```python
from build123d import *

# Parameters (mm, degrees)
SKETCH1_R                 = 9.5377
BOSS_EXTRUDE1_DEPTH       = 29.591
SKETCH2_R                 = 3.81
BOSS_EXTRUDE2_DEPTH       = 10.16
SKETCH3_R                 = 1.9939
CUT_EXTRUDE1_DEPTH        = 12.7
SKETCH4_R                 = 8.4836
CUT_EXTRUDE2_DEPTH        = 27.94
FILLET1_R                 = 3.81
F_4_48_TAPPED_HOLE2_D     = 2.3749
F_4_48_TAPPED_HOLE2_DEPTH = 8.89
F_4_48_TAPPED_HOLE2_TIP   = 0.713491942


with BuildPart() as part:
    # Sketch1 → Boss-Extrude1 (new body)
    with BuildSketch(Plane(origin=(0, 0, 0), x_dir=(1, 0, 0), z_dir=(0, 1, 0))):
        with Locations(Location((0, 0, 0), (0, 0, 90))):
            Circle(SKETCH1_R)
    extrude(amount=BOSS_EXTRUDE1_DEPTH)

    # Sketch2 → Boss-Extrude2 (add)
    with BuildSketch(Plane(origin=(0, 29.591, 0), x_dir=(1, 0, 0), z_dir=(0, 1, 0))):
        with Locations(Location((0, 0, 0), (0, 0, 270))):
            Circle(SKETCH2_R)
    extrude(amount=BOSS_EXTRUDE2_DEPTH)

    # Sketch3 → Cut-Extrude1 (cut)
    with BuildSketch(Plane(origin=(0, 39.751, 0), x_dir=(1, 0, 0), z_dir=(0, 1, 0))):
        with Locations(Location((0, 0, 0), (0, 0, 270))):
            Circle(SKETCH3_R)
    extrude(amount=-CUT_EXTRUDE1_DEPTH, mode=Mode.SUBTRACT)

    # Sketch4 → Cut-Extrude2 (cut)
    with BuildSketch(Plane.XZ):
        with Locations(Location((0, 0, 0), (0, 0, 270))):
            Circle(SKETCH4_R)
    extrude(amount=-CUT_EXTRUDE2_DEPTH, mode=Mode.SUBTRACT)

    # Fillet1
    fillet1_edges = [part.edges().sort_by_distance(p)[0] for p in [
        (0, 29.591, -3.81),
    ]]
    fillet(fillet1_edges, radius=FILLET1_R)

    # #4-48 Tapped Hole2
    with Locations(Plane.XY.offset(9.5377)):
        with Locations((0, 35.941)):
            Hole(F_4_48_TAPPED_HOLE2_D / 2, depth=F_4_48_TAPPED_HOLE2_DEPTH)
            with Locations((0, 0, -(F_4_48_TAPPED_HOLE2_DEPTH + F_4_48_TAPPED_HOLE2_TIP / 2))):  # 118° drill point
                Cone(0, F_4_48_TAPPED_HOLE2_D / 2, F_4_48_TAPPED_HOLE2_TIP, mode=Mode.SUBTRACT)


solid = part.part
```
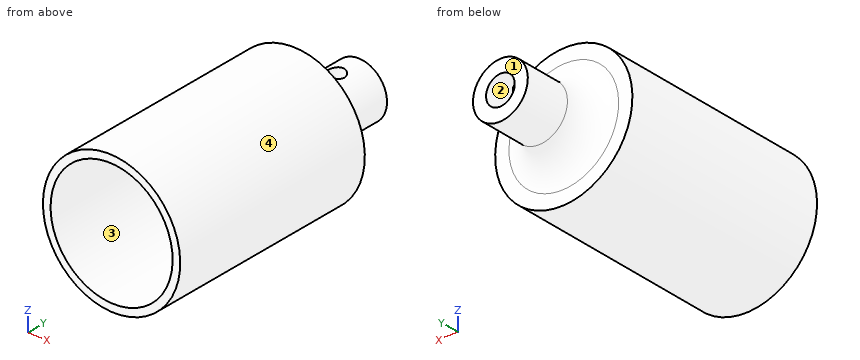
For this review, take the finished solid that the model builds, in its own axes (mm). Face numbers are marked on the shaded views. Give positions to 0.01 mm unless a question says otherwise; leave off trailing zeros. Loops run counter-clockwise (first coordinate to the right, second up) from the corner with the lowest first, then second, coordinate; pieces in that order, holes last. Notation, with made-up numbers: M 85.5,52 L 130.5,52 A34 cw 130.5,84 Z; hole C 81,-39.5 d1. An arc over 180 degrees is marked long. One line per item, written item: value. Start each with the question number.
Q1. Add section B-B (z = 0). Give the boundary of the cut face in (x, y), and give its area (3 significant figures).
Q2. For L1, parallel to X at y = 36.5, z = 0; L2, parallel to Y at x = 3.75, z = 7; L3, parallel to X at y = 31.75, z = 0, list the stretches that pass through material, from the lowest coordinate up.
Q3. Add section D-D (y = 31). Give the boundary of the cut face in (x, z).
Q4. Draft analysis for pull direction Z (two halves, no side actions). For the marked faces 1, 2, 3 and 4, state which applies: released by +Z, released by -Z, zero draft, split by the parting line, or undercut.
Q5. Add section C-C (y = 10). Give the boundary of the cut face in (x, z).
Q6. Clearance check with flat-ended pins moving along their axes: pin 1 Ø4 at (x, y) = (7, 25.5) entering from +Z; pin 2 Ø4 at (x, y) = (-5.5, 18.5) entering from -Z; pin 3 Ø3 at (y, z) = (9.5, 3.5) entering from +X. State where each tip first meets the part, or that it passes through.
Q7. Add section A-A (x = 0). Give the boundary of the cut face in (y, z), and give its area (3 significant figures).
Reply:
1. outline: M -9.54,0 L -8.48,0 L -8.48,27.94 L -1.99,27.94 L -1.99,39.75 L -3.81,39.75 L -3.81,33.4 A3.81 cw -7.62,29.59 L -9.54,29.59 Z; M 1.99,27.94 L 8.48,27.94 L 8.48,0 L 9.54,0 L 9.54,29.59 L 7.62,29.59 A3.81 cw 3.81,33.4 L 3.81,39.75 L 1.99,39.75 Z
1. area: 127 mm²
2. L1: -3.81 to -1.99, 1.99 to 3.81
2. L2: 27.94 to 29.59
2. L3: -4.19 to -1.99, 1.99 to 4.19
3. outline: C 0,0 d9.32; hole C 0,0 d3.99
4. face 1: zero draft
4. face 2: undercut
4. face 3: undercut
4. face 4: split by the parting line
5. outline: C 0,0 d19.08; hole C 0,0 d16.97
6. pin 1: z = 8.12
6. pin 2: z = -8.87
6. pin 3: x = 9.33
7. outline: M 0,-9.54 L 29.59,-9.54 L 29.59,-7.62 A3.81 cw 33.4,-3.81 L 39.75,-3.81 L 39.75,-1.99 L 27.94,-1.99 L 27.94,-8.48 L 0,-8.48 Z; M 0,8.48 L 27.94,8.48 L 27.94,1.99 L 34.75,1.99 L 34.75,3.81 L 33.4,3.81 A3.81 cw 29.59,7.62 L 29.59,9.54 L 0,9.54 Z; M 37.13,1.99 L 39.75,1.99 L 39.75,3.81 L 37.13,3.81 Z
7. area: 123 mm²
